The listing builds one solid part. Answer for the finished solid, in the listing's coordinates (mm). Coordinates: 2 decimals unless noted, no trailing zeros. Order: outer loops, then holes, each group sorted by start corner. A loop starts at its lowest first (then second) coordinate and runs counter-clockwise, first axis right, second up. Notation, with made-up numbers: (12, 20) -> (22, 20) arc R6 ccw to (22, 25) -> close; hole circle Ø9 at (49.25, 13.25). An arc over 180 degrees is marked (long way). Return JSON: item names as keys, results as strings.
from build123d import *

# Parameters (mm, degrees)
SKETCH_1_R      = 34.925
EXTRUDE_1_DEPTH = 21


with BuildPart() as part:
    # 草图1 → 凸台-拉伸1 (new body)
    with BuildSketch(Plane(origin=(0, 0, 0), x_dir=(1, 0, 0), z_dir=(0, 1, 0))):
        with Locations(Location((0, 0, 0), (0, 0, 90))):
            Circle(SKETCH_1_R)
        with BuildLine():
            Line((-2.601341773, 3.505973477), (2.608658475, 3.505973477))
            ThreePointArc((2.608658475, 3.505973477), (3.245054563, 3.242369587), (3.508658453, 2.605973499))
            Line((3.508658453, 2.605973499), (3.508658453, -2.604026749))
            ThreePointArc((3.508658453, -2.604026749), (3.245054563, -3.240422836), (2.608658475, -3.504026727))
            Line((2.608658475, -3.504026727), (-2.601341773, -3.504026727))
            ThreePointArc((-2.601341773, -3.504026727), (-3.23773786, -3.240422836), (-3.501341751, -2.604026749))
            Line((-3.501341751, -2.604026749), (-3.501341751, 2.605973499))
            ThreePointArc((-3.501341751, 2.605973499), (-3.23773786, 3.242369587), (-2.601341773, 3.505973477))
        make_face(mode=Mode.SUBTRACT)
    extrude(amount=EXTRUDE_1_DEPTH)


solid = part.part
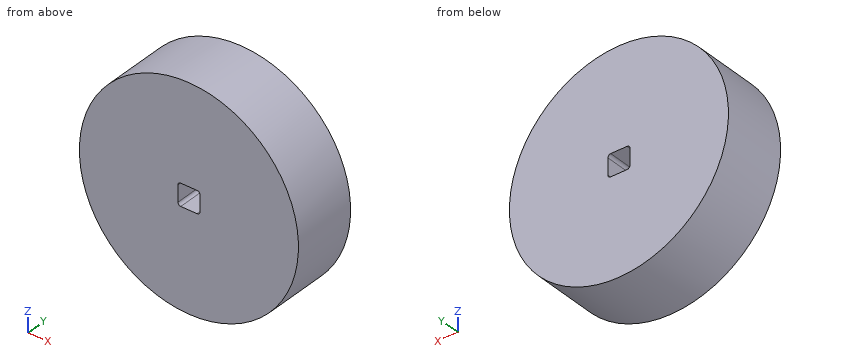
1. The part is cut by section C-C on z = 0. Give the vertices of the cut face in (x, y) (3 decimals), and give its area (3 significant figures).
Answer block:
{"outline": "(-34.925, 0) -> (-3.501, 0) -> (-3.501, 21) -> (-34.925, 21) -> close; (3.509, 0) -> (34.925, 0) -> (34.925, 21) -> (3.509, 21) -> close", "area": "1,320 mm2"}
2. The part is cut by section D-D on x = -19. Give the vertices of the cut face in (y, z).
Answer block:
{"outline": "(0, -29.3) -> (21, -29.3) -> (21, 29.3) -> (0, 29.3) -> close"}
3. Each of these flat-tipped pins is pushed along its axis until it touches: pin 1 Ø12 at (x, y) = (-14, 5) entering from -Z; pin 2 Ø1 at (x, y) = (-16, 10) entering from +Z; pin 3 Ø2.5 at (y, z) = (14, 0.5) entering from -X (3 decimals); pin 4 Ø12 at (x, z) = (-9, -19) entering from -Y. Where does it stop, or does it pass through?
Answer block:
{"pin 1": "stops at z = -34", "pin 2": "stops at z = 31.3", "pin 3": "stops at x = -34.925", "pin 4": "stops at y = 0"}
4. The part is cut by section A-A on y = 9.75. Give the vertices of the cut face in (x, z) (3 decimals), and give its area (3 significant figures).
Answer block:
{"outline": "circle Ø69.85 at (0, 0); hole (-3.501, -2.606) arc R0.9 ccw to (-2.601, -3.506) -> (2.609, -3.506) arc R0.9 ccw to (3.509, -2.606) -> (3.509, 2.604) arc R0.9 ccw to (2.609, 3.504) -> (-2.601, 3.504) arc R0.9 ccw to (-3.501, 2.604) -> close", "area": "3,780 mm2"}
5. The part is cut by section B-B on x = 0. Give the vertices of the cut face in (y, z) (3 decimals).
Answer block:
{"outline": "(0, -34.925) -> (21, -34.925) -> (21, -3.506) -> (0, -3.506) -> close; (0, 3.504) -> (21, 3.504) -> (21, 34.925) -> (0, 34.925) -> close"}
6. Consider line 1 (Z direction, x = -1.5, y = 5.5); line 2 (Z direction, x = -17, y = 7.25); line 3 (Z direction, x = -10, y = 5.75). Determine where each line is inside the solid, lowest interval first. Write a range as from..to.
Answer block:
{"line 1": "z = -34.89..-3.51, 3.5..34.89", "line 2": "z = -30.51..30.51", "line 3": "z = -33.46..33.46"}
